Here's how the part is built. I have some questions about the finished solid (model axes, mm). Face numbers are marked on the shaded views. A direction names the side the tool comes from. Round coordinates to 2 decimals unless told otherwise and drop trailing zeros. Loops run counter-clockwise (first coordinate to the right, second up) from the corner with the lowest first, then second, coordinate; pieces in that order, holes last. Notation, with made-up numbers: M -24,54 L 8,54 A23 cw 8,78 Z; hole C 25,-1.5 d11. An arc over 180 degrees is marked long. One line per question, with ' | ' between items. Start each with the question number.
```python
from build123d import *

# Parameters (mm, degrees)
BOSS_EXTRUDE1_DEPTH = 1.5875
BOSS_EXTRUDE2_DEPTH = 22.225
BOSS_EXTRUDE3_DEPTH = 22.225
BOSS_EXTRUDE4_DEPTH = 1.5875
HOLE1_OUTLINE_R     = 4.826
HOLE1_DEPTH         = 25.4
HOLE2_OUTLINE_R     = 4.826
HOLE2_DEPTH         = 25.4


# Read off the part's stored shape, not the designer's step: Hole1, Hole2
with BuildPart() as part:
    # Sketch4 → Boss-Extrude1 (new body)
    with BuildSketch(Plane(origin=(0, 0, 0), x_dir=(1, 0, 0), z_dir=(0, 1, 0))):
        with BuildLine():
            Line((121.523565154, 38.695091361), (-186.782012798, 38.695091361))
            Line((-186.782012798, 38.695091361), (-186.782012798, 64.095091361))
            Line((-186.782012798, 64.095091361), (130.76840925, 64.095091361))
            Line((130.76840925, 64.095091361), (197.546358654, 8.061738645))
            ThreePointArc((197.546358654, 8.061738645), (199.111720445, -9.830428491), (181.219553308, -11.395790282))
            Line((181.219553308, -11.395790282), (121.523565154, 38.695091361))
        make_face()
    extrude(amount=BOSS_EXTRUDE1_DEPTH)

    # Sketch5 → Boss-Extrude2 (add)
    with BuildSketch(Plane(origin=(0, 1.5875, 0), x_dir=(1, 0, 0), z_dir=(0, 1, 0))):
        with BuildLine():
            Line((-186.782012798, 64.095091361), (-186.782012798, 62.507591361))
            Line((-186.782012798, 62.507591361), (129.436338508, 62.507591361))
            Line((129.436338508, 62.507591361), (129.74798387, 62.878995842))
            Line((129.74798387, 62.878995842), (130.190606494, 62.507591361))
            Line((130.190606494, 62.507591361), (130.768409293, 62.507591361))
            Line((130.768409293, 62.507591361), (130.768409293, 62.022757246))
            Line((130.768409293, 62.022757246), (201.235851163, 2.893552762))
            ThreePointArc((201.235851163, 2.893552762), (199.719327747, 5.7119592), (197.546358654, 8.061738645))
            Line((197.546358654, 8.061738645), (130.76840925, 64.095091361))
            Line((130.76840925, 64.095091361), (-186.782012798, 64.095091361))
        make_face()
    extrude(amount=BOSS_EXTRUDE2_DEPTH)

    # Sketch7 → Boss-Extrude3 (add)
    with BuildSketch(Plane(origin=(0, 1.5875, 0), x_dir=(1, 0, 0), z_dir=(0, 1, 0))):
        with BuildLine():
            Line((-186.782012798, 38.695091361), (-186.782012798, 40.282591361))
            Line((-186.782012798, 40.282591361), (122.10136791, 40.282591361))
            Line((122.10136791, 40.282591361), (186.949896399, -14.131784976))
            ThreePointArc((186.949896399, -14.131784976), (183.910966405, -13.127712138), (181.219553308, -11.395790282))
            Line((181.219553308, -11.395790282), (121.523565154, 38.695091361))
            Line((121.523565154, 38.695091361), (-186.782012798, 38.695091361))
        make_face()
    extrude(amount=BOSS_EXTRUDE3_DEPTH)

    # Sketch8 → Boss-Extrude4 (add)
    with BuildSketch(Plane(origin=(0, 23.8125, 0), x_dir=(1, 0, 0), z_dir=(0, 1, 0))):
        with BuildLine():
            Line((121.523565154, 38.695091361), (-186.782012798, 38.695091361))
            Line((-186.782012798, 38.695091361), (-186.782012798, 64.095091361))
            Line((-186.782012798, 64.095091361), (130.76840925, 64.095091361))
            Line((130.76840925, 64.095091361), (197.546358654, 8.061738645))
            ThreePointArc((197.546358654, 8.061738645), (199.111720445, -9.830428491), (181.219553308, -11.395790282))
            Line((181.219553308, -11.395790282), (121.523565154, 38.695091361))
        make_face()
    extrude(amount=BOSS_EXTRUDE4_DEPTH)

    # Hole1 outline → Hole1 (cut)
    with BuildSketch(Plane(origin=(0, 0, 0), x_dir=(1, 0, 0), z_dir=(0, 1, 0))):
        with Locations((189.382955981, -1.667025818)):
            Circle(HOLE1_OUTLINE_R)
    extrude(amount=HOLE1_DEPTH, mode=Mode.SUBTRACT)

    # Hole2 outline → Hole2 (cut)
    with BuildSketch(Plane(origin=(0, 0, 0), x_dir=(1, 0, 0), z_dir=(0, 1, 0))):
        with Locations((126.145987202, 51.395091361)):
            Circle(HOLE2_OUTLINE_R)
    extrude(amount=HOLE2_DEPTH, mode=Mode.SUBTRACT)


solid = part.part
```
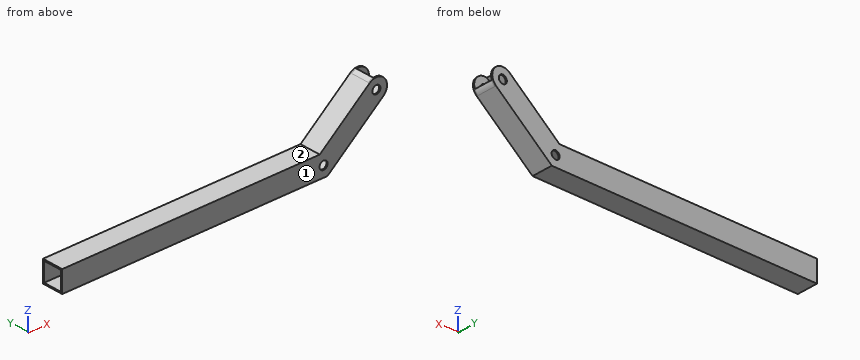
1) I'm going to push flat-ended pins straight in: pin 1 Ø6.5 at (x, y) = (5.5, 12) entering from +Z; pin 2 Ø0.5 at (x, y) = (130.5, 14) entering from +Z; pin 3 Ø7.5 at (x, z) = (189.38, 1.67) entering from -Y; pin 4 Ø3 at (y, z) = (7, -13.5) entering from +X. Where does each tip first touch, or does it pass through?
2) Imagine slicing it at A-A (x = 28.5). Write out the boundary of the cut face in (y, z), then the cut area to 3 significant figures.
3) Imagine slicing it at C-C (z = -24.5). Write out the boundary of the cut face in (x, y), then the cut area to 3 significant figures.
4) Imagine slicing it at B-B (y = 13.5). Write out the boundary of the cut face in (x, z), then the cut area to 3 significant figures.
5) Please list where these lines run through material, in increasing order: L1, parallel to Z at x = 63, y = 14; L2, parallel to Y at x = 166.5, z = -10; L3, parallel to Z at x = 10, y = 24. Write a range as from..to.
6) For the marked faces 1 and 2, which set-ups out of +Z, -Z, +X, -X, +Y, -Y let a thin tool reach every point of the face, with its end or its side?
Results are:
1) pin 1: z = -38.7 | pin 2: z = -30.95 | pin 3: through | pin 4: x = 192.85
2) outline: M 0,-64.1 L 25.4,-64.1 L 25.4,-38.7 L 0,-38.7 Z; hole M 1.59,-62.51 L 23.81,-62.51 L 23.81,-40.28 L 1.59,-40.28 Z | area: 151 mm²
3) outline: M 138.44,0 L 177.96,0 L 177.96,25.4 L 138.44,25.4 Z; hole M 140.91,1.59 L 175.49,1.59 L 175.49,23.81 L 140.91,23.81 Z | area: 235 mm²
4) outline: M -186.78,-64.1 L 130.77,-64.1 L 197.55,-8.06 A12.7 ccw 201.24,-2.89 L 130.77,-62.02 L 130.77,-62.51 L 130.19,-62.51 L 129.75,-62.88 L 129.44,-62.51 L -186.78,-62.51 Z; M -186.78,-40.28 L 122.1,-40.28 L 186.95,14.13 A12.7 ccw 181.22,11.4 L 121.52,-38.7 L -186.78,-38.7 Z | area: 1,270 mm²
5) L1: -64.1..-62.51, -40.28..-38.7 | L2: 0..1.59, 23.81..25.4 | L3: -64.1..-38.7
6) face 1: +Z, -Z, +X, -X, -Y | face 2: +Z, -X, +Y, -Y
